The model under review builds one solid part; all positions refer to its coordinate system, in mm. Face numbers are marked on the shaded views. A direction names the side the tool comes from. Give positions to 0.01 mm unless a question says otherwise; leave off trailing zeros. Order: outer loops, then holes, each group sorted by start corner. A loop starts at its lowest first (then second) coordinate and runs counter-clockwise, first axis right, second up.
```python
from build123d import *

# Parameters (mm, degrees)
ESQUISSE2_R             = 25.041983138
ESQUISSE2_W             = 44.202160672
ESQUISSE2_H             = 23.897916136
ENL_V_MAT_EXTRU_1_DEPTH = 90


with BuildPart() as part:
    # Esquisse1 → Révolution1 (revolve)
    with BuildSketch(Plane.XY, mode=Mode.PRIVATE) as r_volution1_sk:
        Polygon((-45.722988866, 74.192857143), (-5.408703152, 74.192857143), (-5.408703152, 60.592857143), (0, 60.592857143), (0, -16.635714286), (-67.580131723, -2.792857143), (-67.580131723, 5.707142857), (-33.790065862, 5.707142857), (-33.790065862, 62.535714286), (-54.198475628, 62.535714286), align=None)
    revolve(r_volution1_sk.sketch.rotate(Axis((0, 60.592857143, 0), (0, -1, 0)), 270), axis=Axis((0, 60.592857143, 0), (0, -1, 0)))

    # Esquisse2 → Enlèv. mat.-Extru.1 (cut)
    with BuildSketch(Plane(origin=(0, 74.192857143, 0), x_dir=(1, 0, 0), z_dir=(0, 1, 0))):
        with Locations((-79.240458765, 0)):
            Circle(ESQUISSE2_R)
        with Locations((52.10823819, -0.8984179)):
            Rectangle(ESQUISSE2_W, ESQUISSE2_H)
    extrude(amount=-ENL_V_MAT_EXTRU_1_DEPTH, mode=Mode.SUBTRACT)


solid = part.part
```
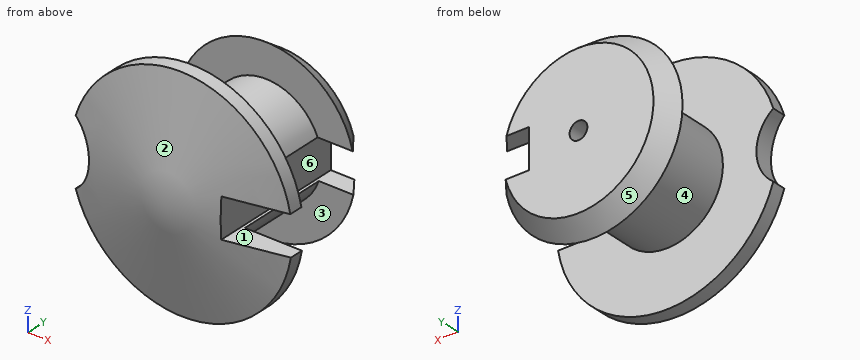
Item 1: For the marked faces 4, 5 and 6, list the 3-axis set-ups (+Z, -Z, +X, -X, +Y, -Y) from which the entire face can be reached by the end or side of a thin tool; tool diameter is ignored.
Values found:
face 4: none
face 5: +Y
face 6: +X, +Y, -Y
Item 2: Take a section at C-C (y = 57.5). Give the boundary of the cut face in (x, z), and give its area (3 significant figures).
Values found:
outline: (30.01, -11.05) - (30.01, 12.85) - (31.25, 12.85) arc R33.79 ccw (long way) to (31.93, -11.05) - close
area: 3,510 mm2
Item 3: Take a section at A-A (y = -1). Give the boundary of the cut face in (x, z).
Values found:
outline: (-64.48, -20.23) arc R67.58 ccw to (66.67, -11.05) - (30.01, -11.05) - (30.01, 12.85) - (66.35, 12.85) arc R67.58 ccw to (-64.48, 20.23) arc R25.04 cw to start
Item 4: Draft analysis for pull direction Z (two halves, no side actions). For the marked faces 1, 2 and 3, state which applies: released by +Z, released by -Z, zero draft, split by the parting line, or undercut.
Values found:
face 1: undercut
face 2: split by the parting line
face 3: zero draft
Item 5: Clearance check with flat-ended pins moving along their axes: pin 1 Ø2 at (y, z) = (20, -17) entering from +X; pin 2 Ø3 at (x, z) = (-43.5, -27) entering from +Y; pin 3 Ø12 at (y, z) = (2.5, -49) entering from -X; pin 4 Ø18.5 at (x, y) = (44.5, 49.5) entering from +Z. State where each tip first meets the part, or that it passes through.
Values found:
pin 1: stops at x = 29.76
pin 2: stops at y = 68.73
pin 3: stops at x = -52.14
pin 4: passes through
Item 6: Take a section at B-B (x = 47.5). Give the number of separate pieces and of enclosed holes in the cut face, and give its area (3 significant figures).
Values found:
separate pieces: 4
enclosed holes: 0
area: 885 mm2
Item 7: For line 1 (X direction, y = 67.5, z = 0); line 2 (Z direction, x = -58, y = 0.5); line 3 (Y direction, x = -43, z = -23), list the stretches that pass through material, from the lowest coordinate up.
Values found:
line 1: x = -50.59 to -5.41, 5.41 to 30.01
line 2: z = -34.69 to -13.26, 13.26 to 34.69
line 3: y = -6.65 to 5.71, 62.54 to 70.01
